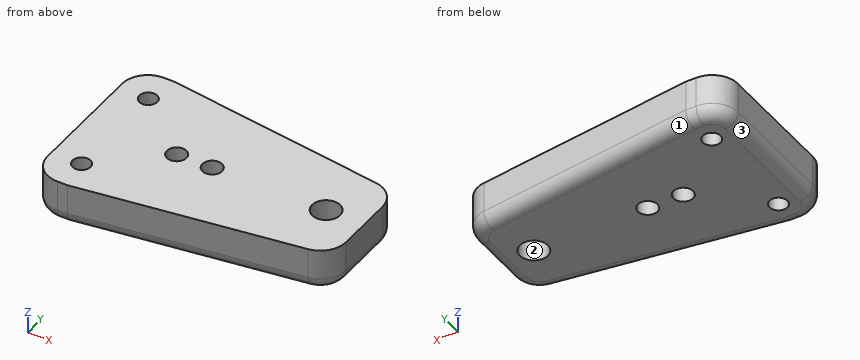
from build123d import *

# Parameters (mm, degrees)
SKETCH1_R            = 2.0828
SKETCH1_R_2          = 3.2639
BASE_EXTRUDE_DEPTH   = 10
SKETCH3_R            = 2.285
HOLES_TO_CLAMP_DEPTH = 11
FILLET2_R            = 3


with BuildPart() as part:
    # Sketch1 → Base-Extrude (new body)
    with BuildSketch(Plane.XY):
        with BuildLine():
            Line((-90.124126187, 20), (-87.749643874, 20))
            Line((-87.749643874, 20), (-36.289087581, 12.767690464))
            ThreePointArc((-36.289087581, 12.767690464), (-32.595868705, 10.762436226), (-31.124126187, 6.826082052))
            Line((-31.124126187, 6.826082052), (-31.124126187, -6.826082052))
            ThreePointArc((-31.124126187, -6.826082052), (-32.595868705, -10.762436226), (-36.289087581, -12.767690464))
            Line((-36.289087581, -12.767690464), (-87.749643874, -20))
            Line((-87.749643874, -20), (-90.124126187, -20))
            ThreePointArc((-90.124126187, -20), (-94.366766874, -18.242640687), (-96.124126187, -14))
            Line((-96.124126187, -14), (-96.124126187, 14))
            ThreePointArc((-96.124126187, 14), (-94.366766874, 18.242640687), (-90.124126187, 20))
        make_face()
        with Locations((-89.124126187, 12.525579086)):
            Circle(SKETCH1_R, mode=Mode.SUBTRACT)
        with Locations((-40, 0)):
            Circle(SKETCH1_R_2, mode=Mode.SUBTRACT)
        with Locations((-89.124126187, -12.525579086)):
            Circle(SKETCH1_R, mode=Mode.SUBTRACT)
    extrude(amount=BASE_EXTRUDE_DEPTH)

    # Sketch3 → Holes to Clamp (cut, through all)
    with BuildSketch(Plane.XY.offset(10)):
        with Locations((-66.489576187, 0)):
            Circle(SKETCH3_R)
        with Locations((-74.749576187, 0)):
            Circle(SKETCH3_R)
    extrude(amount=-HOLES_TO_CLAMP_DEPTH, mode=Mode.SUBTRACT)

    # Fillet2
    fillet2_edges = [part.edges().sort_by_distance(p)[0] for p in [
        (-88.93688503, 20, 0),
        (-62.019365727, 16.383845232, 0),
        (-32.595868705, 10.762436226, 0),
        (-31.124126187, 0, 0),
        (-32.595868705, -10.762436226, 0),
        (-62.019365727, -16.383845232, 0),
        (-88.93688503, -20, 0),
        (-94.366766874, -18.242640687, 0),
        (-96.124126187, 0, 0),
        (-94.366766874, 18.242640687, 0),
    ]]
    fillet(fillet2_edges, radius=FILLET2_R)


solid = part.part
Geometry: final body of the model. Coordinates: model frame, mm. Face numbers are marked on the shaded views. Round coordinates to 2 decimals unless told otherwise and drop trailing zeros. Order: outer loops, then holes, each group sorted by start corner. A loop starts at its lowest first (then second) coordinate and runs counter-clockwise, first axis right, second up. Notation, with made-up numbers: (-0.75, 14.5) -> (26.25, 14.5) arc R24 ccw to (26.25, 52.5) -> close; hole circle Ø2 at (37.25, 53.5). An arc over 180 degrees is marked (long way). Put each result on its own line as item: value. Start each with the question number.
Q1. First-contact query: pin 1 (3 mm diameter, centred on y = 8.5, z = 8.5, fed in from +X); pin 2 (2 mm diameter, centred on x = -58.5, z = 4.5, fed in from +Y); pin 3 (5 mm diameter, centred on y = -14, z = 2, fed in from +X). Flat tips, straight axial feed; report the tip coordinate or a pass-through.
Q2. Section B-B on z = 8.75. Return the cut outline in (x, y) (3 decimals).
Q3. Pull-direction query (Y, two-part tool) for the marked faces 1, 2 and 3; classes: +Y half, -Y half, draft (parallel to the pull), parting line (faces both ways), or undercut.
Q4. Section C-C on z = 1.5. Give the number of separate pieces and of enclosed holes in the cut face, and give its area (3 significant figures).
Q5. Line query: probe 1 along X at (y, z) = (1, 1.25); probe 2 along Y at (x, z) = (-40, 5.5); probe 3 along Y at (x, z) = (-91, 5.5). Output: solid intervals per line, ascending.
Q6. Section A-A on y = 0. Return the cut outline in (x, z), and give its area (3 significant figures).
Ans:
1. pin 1: stops at x = -31.13
1. pin 2: stops at y = 16.03
1. pin 3: stops at x = -33.49
2. outline: (-96.124, -14) arc R6 ccw to (-90.124, -20) -> (-87.75, -20) -> (-36.289, -12.768) arc R6 ccw to (-31.124, -6.826) -> (-31.124, 6.826) arc R6 ccw to (-36.289, 12.768) -> (-87.75, 20) -> (-90.124, 20) arc R6 ccw to (-96.124, 14) -> close; hole circle Ø4.166 at (-89.124, -12.526); hole circle Ø4.166 at (-89.124, 12.526); hole circle Ø4.57 at (-74.75, 0); hole circle Ø4.57 at (-66.49, 0); hole circle Ø6.528 at (-40, 0)
3. face 1: +Y half
3. face 2: undercut
3. face 3: draft
4. separate pieces: 1
4. enclosed holes: 5
4. area: 1,950 mm2
5. probe 1: x = -95.56 to -76.8, -72.7 to -68.54, -64.44 to -43.11, -36.89 to -31.69
5. probe 2: y = -13.29 to -3.26, 3.26 to 13.29
5. probe 3: y = -19.94 to -13.43, -11.62 to 11.62, 13.43 to 19.94
6. outline: (-96.12, 3) arc R3 ccw to (-93.12, 0) -> (-77.03, 0) -> (-77.03, 10) -> (-96.12, 10) -> close; (-72.46, 0) -> (-68.77, 0) -> (-68.77, 10) -> (-72.46, 10) -> close; (-64.2, 0) -> (-43.26, 0) -> (-43.26, 10) -> (-64.2, 10) -> close; (-36.74, 0) -> (-34.12, 0) arc R3 ccw to (-31.12, 3) -> (-31.12, 10) -> (-36.74, 10) -> close
6. area: 489 mm2
